Here's how the part is built. I have some questions about the finished solid (model axes, mm). A direction names the side the tool comes from. Coordinates: 2 decimals unless noted, no trailing zeros. Loops run counter-clockwise (first coordinate to the right, second up) from the corner with the lowest first, then second, coordinate; pieces in that order, holes last. Notation, with made-up numbers: (83, -2.5) -> (89, -2.5) arc R29 cw to (89, 27.5) -> close; hole circle Ø4 at (8.5, -10). An arc over 180 degrees is marked (long way). Answer as a JSON object with one key per item and string values. Group by question number.
1) I want a section at A-A (x = 38.5). Write out the boundary of the cut face in (y, z).
2) I'm going to push a flat-ended pin straight in: pin 1 (1.8 mm diameter, centred on x = -56, z = 25, fed in from +Y). Where does the tip first touch, or does it pass through?
3) Which directions (+Z, -Z, +X, -X, +Y, -Y) give clear straight access to the entire face, cutting with the end or side of a thin tool? Please do faces 1 (the cylindrical face through (-57.82, -0.84, 24.9)), 2 (the flat face through (0, -1, -53)).
4) I need wall thicknesses on probe 1 along Z at (x, y) = (38.5, -2.8); probe 2 along X at (y, z) = (-2.65, 24); probe 3 along X at (y, z) = (-3.4, 35). Which ranges of each line are inside material? Lowest first, please. Write a range as [from, to].
5) I want a section at B-B (z = 24). Write out the boundary of the cut face in (x, y), then the cut area to 3 significant figures.
```python
from build123d import *

# Parameters (mm, degrees)
F0_W     = 127
F0_H     = 106
F0_R     = 1.5
F1_DEPTH = 4
F2_R     = 1
F3_R     = 3
F3_R_2   = 1.5
F4_DEPTH = 1.7


with BuildPart() as f1:
    # F0 (on Front) → F1 (new body)
    with BuildSketch(Plane.XZ):
        with Locations((1, 0)):
            Rectangle(F0_W, F0_H)
        with Locations((-21.5, -23)):
            Circle(F0_R, mode=Mode.SUBTRACT)
        with Locations((38.5, -23)):
            Circle(F0_R, mode=Mode.SUBTRACT)
        with Locations((-54.956626, 7)):
            Circle(F0_R, mode=Mode.SUBTRACT)
        with Locations((-40.28926, 7)):
            Circle(F0_R, mode=Mode.SUBTRACT)
        with Locations((-54.956626, 24)):
            Circle(F0_R, mode=Mode.SUBTRACT)
        with Locations((-40.28926, 24)):
            Circle(F0_R, mode=Mode.SUBTRACT)
        with Locations((-17.5, 35)):
            Circle(F0_R, mode=Mode.SUBTRACT)
        with Locations((47.5, 10)):
            Circle(F0_R, mode=Mode.SUBTRACT)
        with Locations((57.5, 10)):
            Circle(F0_R, mode=Mode.SUBTRACT)
        with Locations((38.5, 35)):
            Circle(F0_R, mode=Mode.SUBTRACT)
    extrude(amount=F1_DEPTH)

    # F2
    f2_edges = [f1.edges().sort_by_distance(p)[0] for p in [
        (1, -4, 53),
        (-62.5, -4, 0),
        (64.5, -4, 0),
        (1, -4, -53),
    ]]
    fillet(f2_edges, radius=F2_R)

    # F3 (on face) → F4 (cut)
    with BuildSketch(Plane(origin=(0, 0, 0), x_dir=(-1, 0, 0), z_dir=(0, 1, 0))):
        with Locations((-38.5, -23)):
            Circle(F3_R)
        with Locations((-38.5, -23)):
            Circle(F3_R_2, mode=Mode.SUBTRACT)
        with Locations((-57.5, 10)):
            Circle(F3_R)
        with Locations((-57.5, 10)):
            Circle(F3_R_2, mode=Mode.SUBTRACT)
        with Locations((-47.5, 10)):
            Circle(F3_R)
        with Locations((-47.5, 10)):
            Circle(F3_R_2, mode=Mode.SUBTRACT)
        with Locations((-38.5, 35)):
            Circle(F3_R)
        with Locations((-38.5, 35)):
            Circle(F3_R_2, mode=Mode.SUBTRACT)
        with Locations((17.5, 35)):
            Circle(F3_R)
        with Locations((17.5, 35)):
            Circle(F3_R_2, mode=Mode.SUBTRACT)
        with Locations((40.28926, 24)):
            Circle(F3_R)
        with Locations((40.28926, 24)):
            Circle(F3_R_2, mode=Mode.SUBTRACT)
        with Locations((54.956626, 24)):
            Circle(F3_R)
        with Locations((54.956626, 24)):
            Circle(F3_R_2, mode=Mode.SUBTRACT)
        with Locations((54.956626, 7)):
            Circle(F3_R)
        with Locations((54.956626, 7)):
            Circle(F3_R_2, mode=Mode.SUBTRACT)
        with Locations((40.28926, 7)):
            Circle(F3_R)
        with Locations((40.28926, 7)):
            Circle(F3_R_2, mode=Mode.SUBTRACT)
        with Locations((21.5, -23)):
            Circle(F3_R)
        with Locations((21.5, -23)):
            Circle(F3_R_2, mode=Mode.SUBTRACT)
    extrude(amount=-F4_DEPTH, mode=Mode.SUBTRACT)


solid = f1.part
```
Determined:
{
 "1": {"outline": "(-4, -52) arc R1 ccw to (-3, -53) -> (0, -53) -> (0, -26) -> (-1.7, -26) -> (-1.7, -24.5) -> (-4, -24.5) -> close; (-4, -21.5) -> (-1.7, -21.5) -> (-1.7, -20) -> (0, -20) -> (0, 32) -> (-1.7, 32) -> (-1.7, 33.5) -> (-4, 33.5) -> close; (-4, 36.5) -> (-1.7, 36.5) -> (-1.7, 38) -> (0, 38) -> (0, 53) -> (-3, 53) arc R1 ccw to (-4, 52) -> close"},
 "2": {"pin 1": "y = -1.7"},
 "3": {"face 1": "+Y", "face 2": "-Z, +X, -X, +Y, -Y"},
 "4": {"probe 1": "[-53, -24.5], [-21.5, 33.5], [36.5, 53]", "probe 2": "[-62.5, -56.46], [-53.46, -41.79], [-38.79, 64.5]", "probe 3": "[-62.42, -19], [-16, 37], [40, 64.42]"},
 "5": {"outline": "(-62.5, -3) arc R1 ccw to (-61.5, -4) -> (-56.46, -4) -> (-56.46, -1.7) -> (-57.96, -1.7) -> (-57.96, 0) -> (-62.5, 0) -> close; (-53.46, -4) -> (-41.79, -4) -> (-41.79, -1.7) -> (-43.29, -1.7) -> (-43.29, 0) -> (-51.96, 0) -> (-51.96, -1.7) -> (-53.46, -1.7) -> close; (-38.79, -4) -> (63.5, -4) arc R1 ccw to (64.5, -3) -> (64.5, 0) -> (-37.29, 0) -> (-37.29, -1.7) -> (-38.79, -1.7) -> close", "area": "473 mm^2"}
}
